The drawing under review shows one solid part. Ordinate dimensions are in mm from its lowest x, y, z. Round coordinates to 2 decimals unless told otherwise and drop trailing zeros. Order: outer loops, then holes, each group sorted by start corner. A loop starts at its lowest first (then second) coordinate and runs counter-clockwise, first axis right, second up. Notation, with made-up numbers: (46, 46) - (62, 46) arc R16 ccw to (62, 52) - close; hole circle Ø6 at (54.5, 68). An arc over 180 degrees is marked (long way). Answer as a JSON object with one key per item and string values. Group by question number.
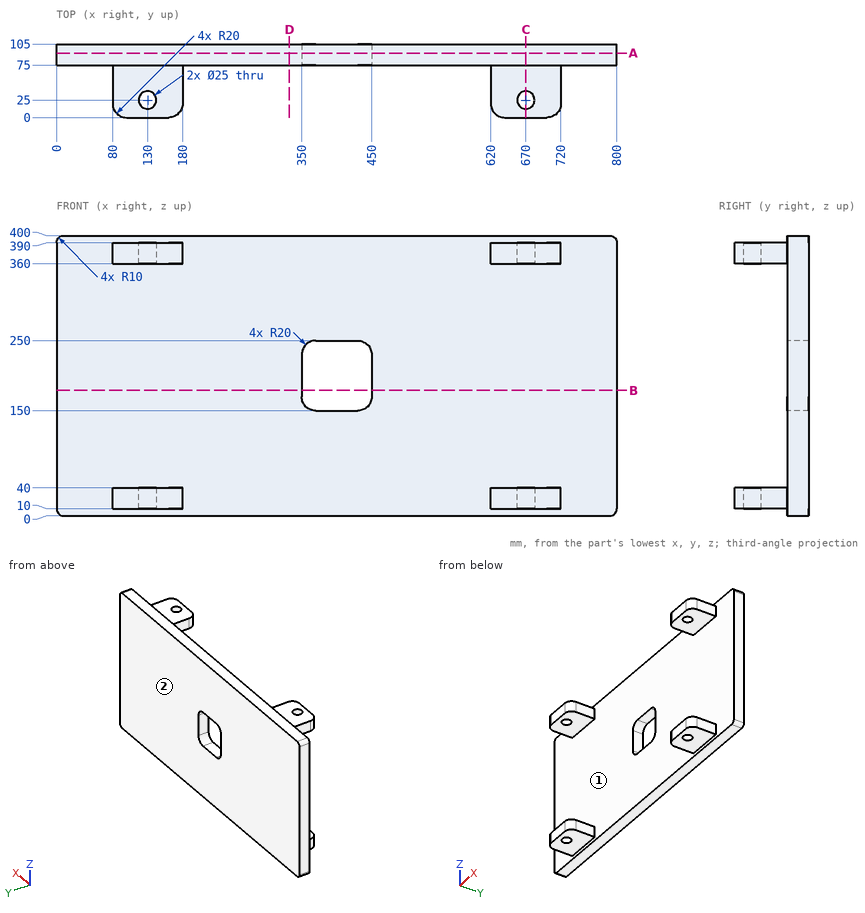
1. Take a section at A-A, the plane y = 92. Give the boundary of the cut face in (x, z), then the cut area to 3 significant figures.
2. To check wall thickness, follow line 1 (Y direction, x = 130, z = 28); line 2 (Z direction, x = 150, y = 45.5); line 3 (X direction, y = 16, z = 372). State the ranges of each line that lie inside material, in increasing order. Write a range as from..to.
3. Clearance check with flat-ended pins moving along their axes: P1, Ø5, axis at x = 103.5, z = 280.5, coming from the -Y side; P2, Ø24, axis at y = 56.5, z = 371, coming from the +X side; P3, Ø15, axis at y = 54.5, z = 22.5, coming from the -X side. State where each tip first meets the part, or that it passes through.
4. Take a section at B-B, the plane z = 179. Give the boundary of the cut face in (x, y), then the cut area to 3 significant figures.
5. Take a section at D-D, the plane x = 332.5. Give the boundary of the cut face in (y, z), then the cut area to 3 significant figures.
6. Mouldability with a two-part tool opening along Z and no side actions: class the marked faces 1 and 2 as pulls with the +Z half, pulls with the -Z half, needs draft (parallel to the pull), parting line crosses it, or undercut.
7. Take a section at C-C, the plane x = 670. Give the boundary of the cut face in (y, z), then the cut area to 3 significant figures.
Response values:
{
 "1": {"outline": "(0, 10) arc R10 ccw to (10, 0) - (790, 0) arc R10 ccw to (800, 10) - (800, 390) arc R10 ccw to (790, 400) - (10, 400) arc R10 ccw to (0, 390) - close; hole (350, 170) arc R20 ccw to (370, 150) - (430, 150) arc R20 ccw to (450, 170) - (450, 230) arc R20 ccw to (430, 250) - (370, 250) arc R20 ccw to (350, 230) - close", "area": "310,000 mm2"},
 "2": {"line 1": "0..12.5, 37.5..105", "line 2": "10..40, 360..390", "line 3": "80.4..121.33, 138.67..179.6, 620.4..661.33, 678.67..719.6"},
 "3": {"P1": "y = 75", "P2": "x = 720", "P3": "x = 80"},
 "4": {"outline": "(0, 75) - (350, 75) - (350, 105) - (0, 105) - close; (450, 75) - (800, 75) - (800, 105) - (450, 105) - close", "area": "21,000 mm2"},
 "5": {"outline": "(75, 0) - (105, 0) - (105, 400) - (75, 400) - close", "area": "12,000 mm2"},
 "6": {"face 1": "undercut", "face 2": "needs draft"},
 "7": {"outline": "(0, 10) - (12.5, 10) - (12.5, 40) - (0, 40) - close; (0, 360) - (12.5, 360) - (12.5, 390) - (0, 390) - close; (37.5, 10) - (75, 10) - (75, 0) - (105, 0) - (105, 400) - (75, 400) - (75, 390) - (37.5, 390) - (37.5, 360) - (75, 360) - (75, 40) - (37.5, 40) - close", "area": "15,000 mm2"}
}
